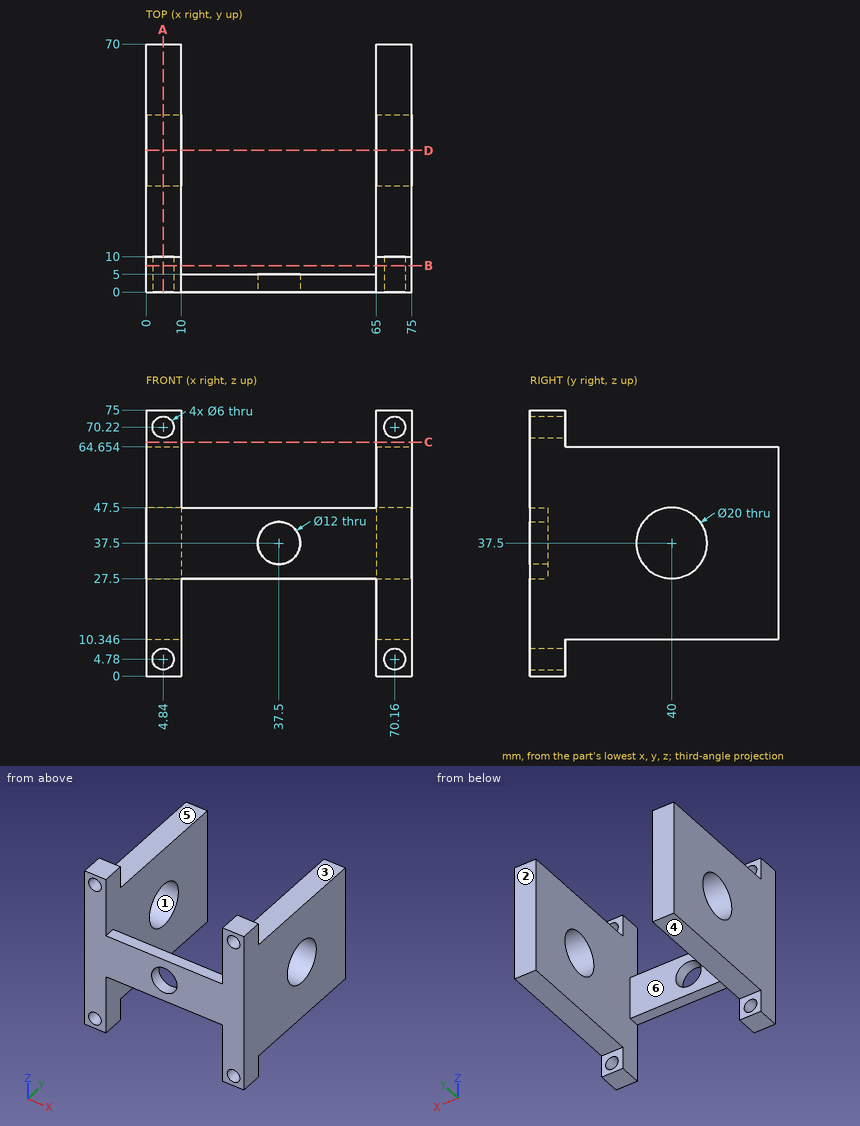
Geometry check sheet. Reference: drawing and pictorial views, mm from the part's lowest x, y, z. A direction names the side the tool comes from. Coordinates: 2 decimals unless noted, no trailing zeros. Write each loop counter-clockwise with the first axis right and the second up, starting at its lowest first coordinate (ties: lowest second). Pieces come first, ordered by that corner, then holes. Notation, with made-up numbers: (80, 19) -> (85, 19) arc R20 cw to (85, 34) -> close; hole circle Ø10 at (-26, 74.25). An arc over 180 degrees is marked (long way). One line per question, with ' | ' between items.
1. Set-up check for the marked faces 4, 5 and 6: record each of +Z, -Z, +X, -X, +Y, -Y from which the full face is reachable in a straight line by a thin tool's end or side.
Answers:
face 4: -Z, +X, -X, +Y | face 5: +Z, +X, -X, +Y | face 6: +Z, -Z, +Y
2. Thickness scan on probe 1 along X at (y, z) = (7.75, 4.78); probe 2 along Y at (x, z) = (3.5, 37.5); probe 3 along X at (y, z) = (33, 51). Record the ranges inside material, lowest first. Write a range as from..to.
Answers:
probe 1: x = 0..1.84, 7.84..10, 65..67.16, 73.16..75 | probe 2: y = 0..30, 50..70 | probe 3: x = 0..10, 65..75
3. Draft check along Y on the marked faces 1, 2 and 3. Enter one of: +Y half, -Y half, draft (parallel to the pull), parting line (faces both ways), or undercut.
Answers:
face 1: undercut | face 2: +Y half | face 3: draft
4. Cross-section at D-D on y = 40. Record the cut outline in (x, z), and give its area (3 significant figures).
Answers:
outline: (0, 10.35) -> (10, 10.35) -> (10, 27.5) -> (0, 27.5) -> close; (0, 47.5) -> (10, 47.5) -> (10, 64.65) -> (0, 64.65) -> close; (65, 10.35) -> (75, 10.35) -> (75, 27.5) -> (65, 27.5) -> close; (65, 47.5) -> (75, 47.5) -> (75, 64.65) -> (65, 64.65) -> close | area: 686 mm²
5. Cross-section at A-A on x = 4.84. Record the cut outline in (y, z), and give its area (3 significant figures).
Answers:
outline: (0, 0) -> (10, 0) -> (10, 1.78) -> (0, 1.78) -> close; (0, 7.78) -> (10, 7.78) -> (10, 10.35) -> (70, 10.35) -> (70, 64.65) -> (10, 64.65) -> (10, 67.22) -> (0, 67.22) -> close; (0, 73.22) -> (10, 73.22) -> (10, 75) -> (0, 75) -> close; hole circle Ø20 at (40, 37.5) | area: 3,570 mm²
6. Cross-section at B-B on y = 7.5. Record the cut outline in (x, z), and give its area (3 significant figures).
Answers:
outline: (0, 0) -> (10, 0) -> (10, 75) -> (0, 75) -> close; (65, 0) -> (75, 0) -> (75, 75) -> (65, 75) -> close; hole circle Ø6 at (4.84, 4.78); hole circle Ø6 at (4.84, 70.22); hole circle Ø6 at (70.16, 4.78); hole circle Ø6 at (70.16, 70.22) | area: 1,390 mm²
7. Cross-section at C-C on z = 66. Record the cut outline in (x, y), and give its area (3 significant figures).
Answers:
outline: (0, 0) -> (10, 0) -> (10, 10) -> (0, 10) -> close; (65, 0) -> (75, 0) -> (75, 10) -> (65, 10) -> close | area: 200 mm²
8. Depth check by flat-ended pin: pin 1 Ø12 at (x, z) = (27, 34) entering from +Y; pin 2 Ø2.5 at (x, y) = (26, 1.5) entering from -Z; pin 3 Ø1 at (x, y) = (64, 60) entering from +Z; pin 4 Ø8 at (x, y) = (2.5, 54.5) entering from -Z. Enter the tip coordinate at first touch or a pass-through.
Answers:
pin 1: stops at y = 5 | pin 2: stops at z = 27.5 | pin 3: passes through | pin 4: stops at z = 10.35
